from build123d import *

# Parameters (mm, degrees)
SKETCH2_W                                       = 57.5
SKETCH2_H                                       = 57.5
BOSS_EXTRUDE1_DEPTH                             = 4
CUT_EXTRUDE4_DEPTH                              = 2.4
M3_CLEARANCE_HOLE1_D                            = 3.4
CSK_FOR_M3_FLAT_HEAD_MACHINE_SCREW1_D           = 3.4
CSK_FOR_M3_FLAT_HEAD_MACHINE_SCREW1_CSINK_D     = 6.3
CSK_FOR_M3_FLAT_HEAD_MACHINE_SCREW1_CSINK_ANGLE = 90
CSK_FOR_M3_FLAT_HEAD_MACHINE_SCREW2_D           = 3.4
CSK_FOR_M3_FLAT_HEAD_MACHINE_SCREW2_CSINK_D     = 6.3
CSK_FOR_M3_FLAT_HEAD_MACHINE_SCREW2_CSINK_ANGLE = 90
CHAMFER1_SIZE                                   = 5


with BuildPart() as part:
    # Sketch2 → Boss-Extrude1 (new body)
    with BuildSketch(Plane.XY):
        with Locations((28.75, 28.75)):
            Rectangle(SKETCH2_W, SKETCH2_H)
    extrude(amount=BOSS_EXTRUDE1_DEPTH)

    # Sketch12 → Cut-Extrude4 (cut)
    with BuildSketch(Plane.XY):
        Polygon((45, 41.766838493), (47.8, 43.383419246), (47.8, 46.616580754), (45, 48.233161507), (42.2, 46.616580754), (42.2, 43.383419246), align=None)
    extrude(amount=CUT_EXTRUDE4_DEPTH, mode=Mode.SUBTRACT)

    # M3 Clearance Hole1 (through all)
    with Locations(Plane.XY.offset(4)):
        with Locations((45, 45), (-45, 45), (-45, -45), (45, -45)):
            Hole(M3_CLEARANCE_HOLE1_D / 2)

    # CSK for M3 Flat Head Machine Screw1 (through all)
    with Locations(Plane.XY.offset(4)):
        with Locations((0, 50), (0, 0), (48, 0)):
            CounterSinkHole(CSK_FOR_M3_FLAT_HEAD_MACHINE_SCREW1_D / 2, CSK_FOR_M3_FLAT_HEAD_MACHINE_SCREW1_CSINK_D / 2, counter_sink_angle=CSK_FOR_M3_FLAT_HEAD_MACHINE_SCREW1_CSINK_ANGLE)

    # CSK for M3 Flat Head Machine Screw2 (through all)
    with Locations(Plane(origin=(0, 0, 0), x_dir=(-1, 0, 0), z_dir=(0, 0, -1))):
        with Locations((-24, 54), (-40, 54)):
            CounterSinkHole(CSK_FOR_M3_FLAT_HEAD_MACHINE_SCREW2_D / 2, CSK_FOR_M3_FLAT_HEAD_MACHINE_SCREW2_CSINK_D / 2, counter_sink_angle=CSK_FOR_M3_FLAT_HEAD_MACHINE_SCREW2_CSINK_ANGLE)

    # Chamfer1
    chamfer1_edges = [part.edges().sort_by_distance(p)[0] for p in [
        (57.5, 57.5, 2),
    ]]
    chamfer(chamfer1_edges, length=CHAMFER1_SIZE)

    # Mirror1: part across plane


with BuildPart() as part_1:
    add(part.part)
    add(part.part.mirror(Plane(origin=(0, 0, 0), x_dir=(0, 0, 1), z_dir=(0, -1, 0))))

    # Mirror2: part across plane


with BuildPart() as part_2:
    add(part_1.part)
    add(part_1.part.mirror(Plane(origin=(0, 0, 0), x_dir=(0, 0, 1), z_dir=(1, 0, 0))))


solid = part_2.part
Here's how the part is built. I have some questions about the finished solid (model axes, mm). A direction names the side the tool comes from. Give positions to 0.01 mm unless a question says otherwise; leave off trailing zeros. Loops run counter-clockwise (first coordinate to the right, second up) from the corner with the lowest first, then second, coordinate; pieces in that order, holes last. Notation, with made-up numbers: (76.25, 29) -> (110.25, 29) arc R26 cw to (110.25, 54) -> close; hole circle Ø8 at (54.25, -9.75). An arc over 180 degrees is marked (long way). Answer as a JSON object with one key per item and string values. Group by question number.
Item 1: Imagine slicing it at B-B on y = 45. Write out the boundary of the cut face in (x, z).
Item 2: I need wall thicknesses on L1, parallel to Y at x = 24, z = 2.9; L2, parallel to Y at x = 45, z = 3.2; L3, parallel to X at y = 54, z = 2.9. Which ranges of each line are inside material? Lowest first, please.
Item 3: Thinking about a two-plate mould opening in Y: for faces 3 (the flat face through (14, -1, 4)), 4 (the cylindrical face through (25.57, 53.35, 2.74)), 5 (the flat face through (1, -57.5, 2)), which applies, pulls with the +Y half, pulls with the -Y half, needs draft (parallel to the pull), parting line crosses it, or undercut?
Item 4: Will this pin go through, and if not, where does the flat tip stop? pin 1 (2.5 mm diameter, centred on x = 45, y = -45, fed in from +Z).
Item 5: Imagine slicing it at C-C on y = 0. Write out the boundary of the cut face in (x, z).
Item 6: Imagine slicing it at A-A on x = 40. Write out the boundary of the cut face in (y, z), then the cut area to 3 significant figures.
Item 7: On a 3-axis mill with a long thin cutter (end or side, diameter ignored), from which of +Z, -Z, +X, -X, +Y, -Y can I reach the whole of each face in a straight line? I mean faces 1 (the cylindrical face through (49.7, -0.07, 1.26)), 2 (the flat face through (-43.7, -43.6, 2.4)). Say none if no direction works.
Answer list:
{
 "1": {"outline": "(-57.5, 0) -> (-47.8, 0) -> (-47.8, 2.4) -> (-46.7, 2.4) -> (-46.7, 4) -> (-57.5, 4) -> close; (-43.3, 2.4) -> (-42.2, 2.4) -> (-42.2, 0) -> (42.2, 0) -> (42.2, 2.4) -> (43.3, 2.4) -> (43.3, 4) -> (-43.3, 4) -> close; (46.7, 2.4) -> (47.8, 2.4) -> (47.8, 0) -> (57.5, 0) -> (57.5, 4) -> (46.7, 4) -> close"},
 "2": {"L1": "y = -57.5 to -55.7, -52.3 to 52.3, 55.7 to 57.5", "L2": "y = -57.5 to -46.7, -43.3 to 43.3, 46.7 to 57.5", "L3": "x = -56 to -41.7, -38.3 to -25.7, -22.3 to 22.3, 25.7 to 38.3, 41.7 to 56"},
 "3": {"face 3": "needs draft", "face 4": "undercut", "face 5": "pulls with the -Y half"},
 "4": {"pin 1": "passes through"},
 "5": {"outline": "(-57.5, 0) -> (-49.7, 0) -> (-49.7, 2.55) -> (-51.15, 4) -> (-57.5, 4) -> close; (-46.3, 0) -> (-1.7, 0) -> (-1.7, 2.55) -> (-3.15, 4) -> (-44.85, 4) -> (-46.3, 2.55) -> close; (1.7, 0) -> (46.3, 0) -> (46.3, 2.55) -> (44.85, 4) -> (3.15, 4) -> (1.7, 2.55) -> close; (49.7, 0) -> (57.5, 0) -> (57.5, 4) -> (51.15, 4) -> (49.7, 2.55) -> close"},
 "6": {"outline": "(-57.5, 0) -> (-57.15, 0) -> (-55.7, 1.45) -> (-55.7, 4) -> (-57.5, 4) -> close; (-52.3, 1.45) -> (-50.85, 0) -> (50.85, 0) -> (52.3, 1.45) -> (52.3, 4) -> (-52.3, 4) -> close; (55.7, 1.45) -> (57.15, 0) -> (57.5, 0) -> (57.5, 4) -> (55.7, 4) -> close", "area": "429 mm2"},
 "7": {"face 1": "+Z, -Z", "face 2": "-Z"}
}
